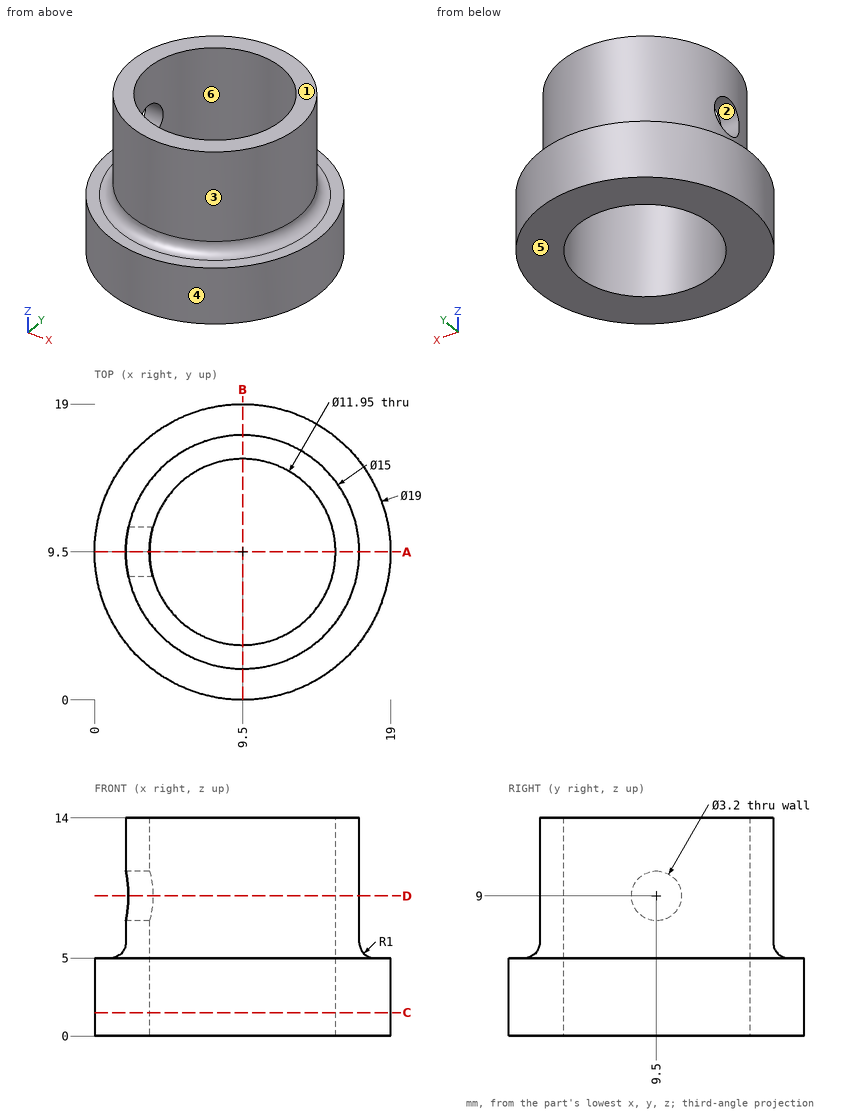
Part print with two shaded views. Sizes in mm from the minimum x, y, z corner. A direction names the side the tool comes from. Coordinates: 2 decimals unless noted, no trailing zeros. Loops run counter-clockwise (first coordinate to the right, second up) from the corner with the lowest first, then second, coordinate; pieces in that order, holes last. Notation, with made-up numbers: M 72.5,35 L 77.5,35 A10 ccw 77.5,42 Z; hole C 14,23 d7. An arc over 180 degrees is marked long. Use CSV: the item, a comma, the result in double quotes. Start each with the question number.
1. Band-saw the part on B-B, the plane x = 9.5. List the corners of the cut face in (y, z) (3 decimals), then the cut area to 3 significant figures.
2. Flat gauge pins, fed straight in: pin 1 (4 mm diameter, centred on x = 10.5, z = 4.5, fed in from -Y); pin 2 (1.5 mm diameter, centred on y = 12.5, z = 7.5, fed in from +X); pin 3 (6 mm diameter, centred on x = 15, z = 2, fed in from +Y); pin 4 (5 mm diameter, centred on y = 9.5, z = 9, fed in from -X). Where does each tip first touch, or does it go through?
3. Band-saw the part on D-D, the plane z = 9. List the corners of the cut face in (x, y) (3 decimals), then the cut area to 3 significant figures.
4. Band-saw the part on A-A, the plane y = 9.5. List the corners of the cut face in (x, z) (3 decimals).
5. Probe probe 1 along Y at (x, z) = (9.5, 8) (3 decimals); probe 2 along Y at (x, z) = (4.5, 10). List the from-to ranges inside material, lowest first. Write a range as [from, to].
6. Band-saw the part on C-C, the plane z = 1.5. List the corners of the cut face in (x, y) (3 decimals).
7. Tool access for the marked faces 1, 2 and 3: list every direction of +Z, -Z, +X, -X, +Y, -Y with a clear straight run to the whole face (end or side of a thin tool).
8. Two-plate mould, pull along Y, no slides. Class the marked faces 4, 5 and 6: pulls with the +Y half, pulls with the -Y half, needs draft (parallel to the pull), parting line crosses it, or undercut.
Entries:
1,outline,"M 0,0 L 3.525,0 L 3.525,14 L 2,14 L 2,6 A1 cw 1,5 L 0,5 Z; M 15.475,0 L 19,0 L 19,5 L 18,5 A1 cw 17,6 L 17,14 L 15.475,14 Z"
1,area,"63.1 mm2"
2,pin 1,"stops at y = 0"
2,pin 2,"stops at x = 16.65"
2,pin 3,"stops at y = 18.67"
2,pin 4,"stops at x = 2"
3,outline,"M 2.173,7.9 A7.5 ccw long 2.173,11.1 L 3.743,11.1 A5.975 cw long 3.743,7.9 Z"
3,area,"59.6 mm2"
4,outline,"M 0,0 L 3.525,0 L 3.525,7.4 L 2,7.4 L 2,6 A1 cw 1,5 L 0,5 Z; M 2,10.6 L 3.525,10.6 L 3.525,14 L 2,14 Z; M 15.475,0 L 19,0 L 19,5 L 18,5 A1 cw 17,6 L 17,14 L 15.475,14 Z"
5,probe 1,"y = [2, 3.525], [15.475, 17]"
5,probe 2,"y = [3.91, 6.23], [12.77, 15.09]"
6,outline,"C 9.5,9.5 d19; hole C 9.5,9.5 d11.95"
7,face 1,"+Z, +X, -X, +Y, -Y"
7,face 2,"-X"
7,face 3,"+Z"
8,face 4,"parting line crosses it"
8,face 5,"needs draft"
8,face 6,"undercut"
